Input: part model. Units: mm. Frame: model coordinates. A direction names the side the tool comes from. Round coordinates to 2 decimals unless told otherwise and drop trailing zeros. Loops run counter-clockwise (first coordinate to the right, second up) from the corner with the lowest first, then second, coordinate; pieces in that order, holes last. Notation, with made-up numbers: (-5, 84) -> (16, 84) arc R20 ccw to (16, 89) -> close; hole circle Ø9 at (32.25, -22). An arc over 180 degrees is marked (long way). One line per question, with ' | ' between items. Start each with the question number.
Q1. Cut plane A-A on z = -17.5. Return loops of the section in (x, y), and give its area (3 significant figures).
Q2. Cut plane D-D on z = -9.5. Return loops of the section in (x, y), and give its area (3 significant figures).
Q3. Mould query, pull axis Y, two halves, no side actions, for faces 1 (the face through (62.61, 0.54, -24.68)), 2 (the face through (63, 65.953, -29)), 3 (the face through (63, 36, 0)). Classes: pulls with the +Y half, pulls with the -Y half, needs draft (parallel to the pull), parting line crosses it, or undercut.
Q4. Access query for faces 4 (the face through (63, -41.743, -10)), 5 (the face through (63, 56, -19.304)), 6 (the face through (63, -61.047, -29)). Directions: +Z, -Z, +X, -X, +Y, -Y. A direction counts if a zero-diameter tool reaches every point of the face in a straight line with its end or side. Return the directions, or none.
Q5. Contact query for flat-ended pins moving along their axis: P1, Ø9.5, axis at x = 73, y = -47.5, coming from the +Z side; P2, Ø1, axis at x = 90, z = -13.5, coming from the -Y side; P3, Ø15.5, axis at x = 75, z = -6.5, coming from the +Y side. Output: stop coordinate, or through.
Q6. Cut plane C-C on y = 0. Return loops of the section in (x, z).
Q7. Cut plane B-B on x = 41. Return loops of the section in (y, z).
Q8. Material intervals for L1, parallel to Z at x = 95, y = 48; L2, parallel to Y at x = 108.5, z = -21.5; L3, parallel to Y at x = 29.5, z = -5, sorted ascending.
from build123d import *

# Parameters (mm, degrees)
F1_DEPTH = 127


with BuildPart() as f1:
    # F0 (on Right) → F1 (new body)
    with BuildSketch(Plane.YZ):
        with BuildLine():
            Line((-41.742593, -19.304), (-61.046593, -19.304))
            Line((-61.046593, -19.304), (-61.046593, -38.608))
            Line((-61.046593, -38.608), (65.953407, -38.608))
            Line((65.953407, -38.608), (65.953407, -19.304))
            Line((65.953407, -19.304), (46.649407, -19.304))
            Line((46.649407, -19.304), (46.649407, 0))
            Line((46.649407, 0), (40.045407, 0))
            Line((40.045407, 0), (24.686914, 0))
            ThreePointArc((24.686914, 0), (0, -24.686914), (-24.686914, 0))
            Line((-24.686914, 0), (-35.138593, 0))
            Line((-35.138593, 0), (-41.742593, 0))
            Line((-41.742593, 0), (-41.742593, -19.304))
        make_face()
    extrude(amount=F1_DEPTH)


solid = f1.part
Results:
1) outline: (0, -41.74) -> (127, -41.74) -> (127, -17.41) -> (0, -17.41) -> close; (0, 17.41) -> (127, 17.41) -> (127, 46.65) -> (0, 46.65) -> close | area: 6,800 mm^2
2) outline: (0, -41.74) -> (127, -41.74) -> (127, -22.79) -> (0, -22.79) -> close; (0, 22.79) -> (127, 22.79) -> (127, 46.65) -> (0, 46.65) -> close | area: 5,440 mm^2
3) face 1: undercut | face 2: pulls with the +Y half | face 3: needs draft
4) face 4: +Z, +X, -X, -Y | face 5: +Z, +X, -X, +Y | face 6: +Z, -Z, +X, -X, -Y
5) P1: z = -19.3 | P2: y = -41.74 | P3: y = 46.65
6) outline: (0, -38.61) -> (127, -38.61) -> (127, -24.69) -> (0, -24.69) -> close
7) outline: (-61.05, -38.61) -> (65.95, -38.61) -> (65.95, -19.3) -> (46.65, -19.3) -> (46.65, 0) -> (24.69, 0) arc R24.69 cw to (-24.69, 0) -> (-41.74, 0) -> (-41.74, -19.3) -> (-61.05, -19.3) -> close
8) L1: -38.61 to -19.3 | L2: -61.05 to -12.13, 12.13 to 65.95 | L3: -41.74 to -24.18, 24.18 to 46.65
